Check sheet for the modelled part. Datum: model origin and axes. Units: mm. Coordinates: 2 decimals unless noted, no trailing zeros. Loops run counter-clockwise (first coordinate to the right, second up) from the corner with the lowest first, then second, coordinate; pieces in that order, holes last. Notation, with made-up numbers: (-31.75, 79) - (-10.75, 79) arc R18 ccw to (-10.75, 93) - close; hole circle Ø1 at (67, -6.5). An arc over 180 degrees is marked (long way). Use a Markdown table: item, result. Add a question column.
1) Go/stop test with flat-tipped pins: P1, Ø20, axis at x = 0, y = 83.175, coming from the -Z side; P2, Ø10, axis at x = 59, y = 82.5, coming from the -Z side. Record where each tip stops, or that it passes through.
2) Sectioned sample at A-A, the plane x = 87. Enter the section's corners in (y, z) (3 decimals).
3) Sectioned sample at D-D, the plane x = 3. Enter the section's corners in (y, z) (3 decimals).
4) Thickness scan on line 1 (Y direction, x = 0, z = 2.2) (3 decimals); line 2 (X direction, y = 80, z = 2.7); line 3 (Y direction, x = 85, z = 0.5) (3 decimals). Record the ranges inside material, lowest first.
5) Sectioned sample at B-B, the plane y = 91. Enter the section's corners in (x, z) (3 decimals).
6) Sectioned sample at C-C, the plane z = 0.6. Enter the section's corners in (x, y) (1 decimal), then the cut area to 3 significant figures.
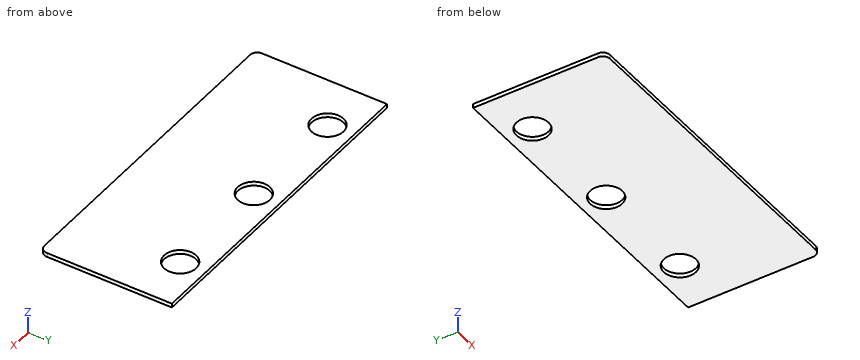
from build123d import *

# Parameters (mm, degrees)
SKETCH1_W           = 254
SKETCH1_H           = 103.175
SKETCH1_R           = 12.5
BOSS_EXTRUDE1_DEPTH = 3.175
FILLET1_R           = 5.55625


with BuildPart() as part:
    # Sketch1 → Boss-Extrude1 (new body)
    with BuildSketch(Plane.XY):
        with Locations((0, 51.5875)):
            Rectangle(SKETCH1_W, SKETCH1_H)
        with Locations((87, 83.175)):
            Circle(SKETCH1_R, mode=Mode.SUBTRACT)
        with Locations((-87, 83.175)):
            Circle(SKETCH1_R, mode=Mode.SUBTRACT)
        with Locations((0, 83.175)):
            Circle(SKETCH1_R, mode=Mode.SUBTRACT)
    extrude(amount=BOSS_EXTRUDE1_DEPTH)

    # Fillet1
    fillet1_edges = [part.edges().sort_by_distance(p)[0] for p in [
        (127, 0, 1.5875),
        (-127, 0, 1.5875),
    ]]
    fillet(fillet1_edges, radius=FILLET1_R)


solid = part.part
Solved:
| question | item | result |
|---|---|---|
| 1 | P1 | passes through |
| 1 | P2 | stops at z = 0 |
| 2 | outline | (0, 0) - (70.675, 0) - (70.675, 3.175) - (0, 3.175) - close; (95.675, 0) - (103.175, 0) - (103.175, 3.175) - (95.675, 3.175) - close |
| 3 | outline | (0, 0) - (71.04, 0) - (71.04, 3.175) - (0, 3.175) - close; (95.31, 0) - (103.175, 0) - (103.175, 3.175) - (95.31, 3.175) - close |
| 4 | line 1 | y = 0 to 70.675, 95.675 to 103.175 |
| 4 | line 2 | x = -127 to -99.09, -74.91 to -12.09, 12.09 to 74.91, 99.09 to 127 |
| 4 | line 3 | y = 0 to 70.836, 95.514 to 103.175 |
| 5 | outline | (-127, 0) - (-96.748, 0) - (-96.748, 3.175) - (-127, 3.175) - close; (-77.252, 0) - (-9.748, 0) - (-9.748, 3.175) - (-77.252, 3.175) - close; (9.748, 0) - (77.252, 0) - (77.252, 3.175) - (9.748, 3.175) - close; (96.748, 0) - (127, 0) - (127, 3.175) - (96.748, 3.175) - close |
| 6 | outline | (-127, 5.6) arc R5.6 ccw to (-121.4, 0) - (121.4, 0) arc R5.6 ccw to (127, 5.6) - (127, 103.2) - (-127, 103.2) - close; hole circle Ø25 at (-87, 83.2); hole circle Ø25 at (0, 83.2); hole circle Ø25 at (87, 83.2) |
| 6 | area | 24,700 mm2 |
